Design review of the part built by this model. Coordinates are the model's own, in mm. A direction names the side the tool comes from. Give positions to 0.01 mm unless a question says otherwise; leave off trailing zeros. Loops run counter-clockwise (first coordinate to the right, second up) from the corner with the lowest first, then second, coordinate; pieces in that order, holes last.
Autodesk Fusion 360 part; units mm, degrees
sketch "Sketch1" plane through (0, 0, 0) normal (0, 0, 1) x (1, 0, 0)
  line L0 (0, 0) -> (11.7, 0)
  line L1 (11.7, 0) -> (11.7, -4)
  line L2 (11.7, -4) -> (0, -4)
  line L3 (0, -4) -> (0, 0)
  line L4 (5.85, 0) -> (5.85, -4) construction
  line L5 (0, -2) -> (11.7, -2) construction
  line L6 (8.05, -3) -> (3.65, -3)
  line L7 (3.65, -3) -> (3.65, -1)
  line L8 (3.65, -1) -> (8.05, -1)
  line L9 (8.05, -1) -> (8.05, -3)
  line L10 (8.05, -3) -> (3.65, -1) construction
  line L11 (3.65, -3) -> (8.05, -1) construction
  line L12 (3.65, -1) -> (5.65, -1)
  line L13 (5.65, -1) -> (5.65, -3)
  line L14 (5.65, -3) -> (3.65, -3)
  line L15 (3.65, -3) -> (3.65, -1)
  point P0 (5.85, -2)
  dimension "d1" = 11.7
  dimension "d2" = 4
  dimension "d3" = 4.4
  dimension "d4" = 2
  dimension "d5" = 2
extrude "Extrude1" add sketch "Sketch1" against normal blind 6.3 contours L0 L1 L2 L3 | L6 L8 L9 L13 | L6 L7 L8 L12 L13 L14 L15
extrude "Extrude2" cut sketch "Sketch1" against normal blind 0.5 contours L6 L8 L9 L13 | L6 L7 L8 L12 L13 L14 L15
extrude "Extrude3" add sketch "Sketch1" along normal blind 1.7 and the other way blind 0.5 contours L6 L7 L8 L12 L13 L14 L15
sketch "Sketch2" plane through (0, 0, -6.3) normal (0, 0, -1) x (1, 0, 0)
  line L0 (11.7, 4) -> (0, 4)
  line L1 (0, 4) -> (0, 0)
  line L2 (0, 0) -> (11.7, 0)
  line L3 (11.7, 0) -> (11.7, 4)
  line L4 (5.85, 4) -> (5.85, 0) construction
  line L5 (0, 2) -> (11.7, 2) construction
  line L6 (10.85, 0) -> (0.85, 0)
  line L7 (0.85, 0) -> (0.85, 4)
  line L8 (0.85, 4) -> (10.85, 4)
  line L9 (10.85, 4) -> (10.85, 0)
  line L10 (10.85, 0) -> (0.85, 4) construction
  line L11 (0.85, 0) -> (10.85, 4) construction
  point P0 (5.85, 2)
  dimension "d13" = 10
  dimension "d14" = 4
extrude "Extrude4" cut sketch "Sketch2" against normal blind 0.5 contours L0 L2 L6 L7 L8 L9
Q1. Draft analysis for pull direction X (two halves, no side actions). For faces 5 (the face through (6, -2, -5.8)), 6 (the face through (11.7, -2, -3)), 7 (the face through (11, -2, -6.3)), state which applies: pulls with the +X half, pulls with the -X half, needs draft (parallel to the pull), parting line crosses it, or undercut.
Results:
face 5: undercut
face 6: pulls with the +X half
face 7: needs draft
Q2. Take a section at D-D (y = -1.6). Give the boundary of the cut face in (x, z).
Results:
outline: (0, -6.3) - (0.85, -6.3) - (0.85, -5.8) - (10.85, -5.8) - (10.85, -6.3) - (11.7, -6.3) - (11.7, 0) - (8.05, 0) - (8.05, -0.5) - (5.65, -0.5) - (5.65, 1.7) - (3.65, 1.7) - (3.65, 0) - (0, 0) - close
Q3. Take a section at C-C (z = 0.25). Give the boundary of the cut face in (x, y), plus the area to 3 significant figures.
Results:
outline: (3.65, -3) - (5.65, -3) - (5.65, -1) - (3.65, -1) - close
area: 4.00 mm2
Q4. Insertion check: pin 1 (2 mm diameter, centred on x = 5, y = -1.5, fed in from -Z); pin 2 (0.8 mm diameter, centred on x = 5, z = 0.5, fed in from -Y); pin 3 (0.8 mm diameter, centred on y = -1.5, z = 0.5, fed in from -X). Each pin has a flat end and moves straight along its axis. Give the tip position at first contact, or say it passes through.
Results:
pin 1: stops at z = -5.8
pin 2: stops at y = -3
pin 3: stops at x = 3.65
Q5. Take a section at B-B (x = 4.5). Give the boundary of the cut face in (y, z).
Results:
outline: (-4, -5.8) - (0, -5.8) - (0, 0) - (-1, 0) - (-1, 1.7) - (-3, 1.7) - (-3, 0) - (-4, 0) - close
Q6. Tool access review of faces 1 (the face through (7, -2, -0.5)), 2 (the face through (5, -3, 1)), 3 (the face through (5, -1, 1)), 4 (the face through (3.65, -2, 1)): name each direction out of +Z, -Z, +X, -X, +Y, -Y from which nothing blocks a thin tool from reaching the whole face with its end or side.
Results:
face 1: +Z
face 2: +Z, +X, -X, -Y
face 3: +Z, +X, -X, +Y
face 4: +Z, -X, +Y, -Y
Q7. Wall thickness on line 1 (X direction, y = -2.35, z = -6); line 2 (Z direction, x = 8.75, y = -1.95); line 3 (Z direction, x = 6, y = -1.8): over which ranges is each line inside the solid? List them lowest first.
Results:
line 1: x = 0 to 0.85, 10.85 to 11.7
line 2: z = -5.8 to 0
line 3: z = -5.8 to -0.5
Q8. Take a section at A-A (y = -3.6). Give the boundary of the cut face in (x, z).
Results:
outline: (0, -6.3) - (0.85, -6.3) - (0.85, -5.8) - (10.85, -5.8) - (10.85, -6.3) - (11.7, -6.3) - (11.7, 0) - (0, 0) - close
